```python
from build123d import *

# Parameters (mm, degrees)
CHAFL_N2_SIZE         = 0.3
CHAFL_N2_SIZE2        = 0.212132034
CHAFL_N3_SIZE         = 0.3
CORTAR_EXTRUIR2_DEPTH = 1


with BuildPart() as part:
    # Croquis1 → Revolución1 (revolve)
    with BuildSketch(Plane.XY, mode=Mode.PRIVATE) as revoluci_n1_sk:
        Polygon((0, 0), (5.1, 0), (2.5, -2.6), (2.5, -12), (0, -12), align=None)
    revolve(revoluci_n1_sk.sketch.rotate(Axis((0, 0, 0), (0, -1, 0)), 90), axis=Axis((0, 0, 0), (0, -1, 0)))

    # Chaflán2
    chafl_n2_edges = [part.edges().sort_by_distance(p)[0] for p in [
        (0, 0, -5.1),
    ]]
    chafl_n2_side = [part.faces().sort_by_distance(p)[0] for p in [
        (0, -1.3, -3.8),
    ]]
    chamfer(chafl_n2_edges, length=CHAFL_N2_SIZE, length2=CHAFL_N2_SIZE2, reference=chafl_n2_side[0])

    # Chaflán3
    chafl_n3_edges = [part.edges().sort_by_distance(p)[0] for p in [
        (0, -12, -2.5),
    ]]
    chamfer(chafl_n3_edges, length=CHAFL_N3_SIZE)

    # Croquis3 → Cortar-Extruir2 (cut)
    with BuildSketch(Plane(origin=(0, 0, 0), x_dir=(1, 0, 0), z_dir=(0, 1, 0))):
        Polygon((-0.721687836, 1.25), (-1.443375673, 0), (-0.721687836, -1.25), (0.721687836, -1.25), (1.443375673, 0), (0.721687836, 1.25), align=None)
    extrude(amount=-CORTAR_EXTRUIR2_DEPTH, mode=Mode.SUBTRACT)


solid = part.part
```
Here's how the part is built. I have some questions about the finished solid (model axes, mm). A direction names the side the tool comes from. Coordinates: 2 decimals unless noted, no trailing zeros. Order: outer loops, then holes, each group sorted by start corner. A loop starts at its lowest first (then second) coordinate and runs counter-clockwise, first axis right, second up.
Item 1: I need wall thicknesses on probe 1 along Z at (x, y) = (2, -8.75); probe 2 along Y at (x, z) = (1.5, 4.25); probe 3 along Y at (x, z) = (-0.75, -1). Which ranges of each line are inside material? Lowest first, please.
Response values:
probe 1: z = -1.5 to 1.5
probe 2: y = -0.59 to 0
probe 3: y = -12 to -1
Item 2: Which directions (+Z, -Z, +X, -X, +Y, -Y) give clear straight access to the entire face, cutting with the end or side of a thin tool? Please do faces 1 (the face through (-1.08, -0.49, -0.63)), 2 (the face through (-0.1, -7.2, -2.5)), 3 (the face through (0, -12, 0)).
Response values:
face 1: +Y
face 2: -Y
face 3: +Z, -Z, +X, -X, -Y
Item 3: Thinking about a two-plate mould opening in X: for faces 4 (the face through (1.59, -2.48, -2.08)), 5 (the face through (1.08, -0.49, 0.63)), 6 (the face through (1, 0, 1.2)), which applies, pulls with the +X half, pulls with the -X half, needs draft (parallel to the pull), parting line crosses it, or undercut?
Response values:
face 4: parting line crosses it
face 5: undercut
face 6: needs draft
Item 4: I'm going to push flat-ended pins straight in: pin 1 Ø1.5 at (y, z) = (-4.5, -0.5) entering from +X; pin 2 Ø1.5 at (y, z) = (-8, -2) entering from -X; pin 3 Ø3 at (x, y) = (2, -8.5) entering from +Z. Where does each tip first touch, or does it pass through?
Response values:
pin 1: stops at x = 2.5
pin 2: stops at x = -2.17
pin 3: stops at z = 2.45
Item 5: If we section it at A-A, the plane y = -8: List the corners of the cut face in (x, z) for me, then the cut area to 3 significant figures.
Response values:
outline: circle Ø5 at (0, 0)
area: 19.6 mm2
